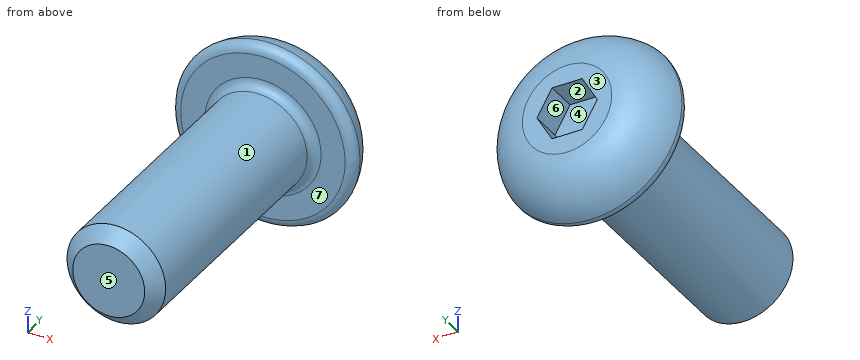
from build123d import *

# Parameters (mm, degrees)
SKETCH2_R           = 1.7526
BOSS_EXTRUDE1_DEPTH = 9.525
CUT_EXTRUDE1_DEPTH  = 1.1176
CHAMFER1_SIZE       = 0.47244
FILLET1_R           = 0.316308646


with BuildPart() as part:
    # Sketch1 → Revolve1 (revolve)
    with BuildSketch(Plane.XY):
        with BuildLine():
            Line((1.5875, 1.8542), (0, 1.8542))
            Line((0, 1.8542), (0, 0))
            Line((0, 0), (3.270560013, 0))
            ThreePointArc((3.270560013, 0), (2.787047666, 1.252073146), (1.5875, 1.8542))
        make_face()
    revolve(axis=Axis((0, 1.8542, 0), (0, -1, 0)))

    # Sketch2 → Boss-Extrude1 (add)
    with BuildSketch(Plane.XZ):
        Circle(SKETCH2_R)
    extrude(amount=BOSS_EXTRUDE1_DEPTH)

    # Sketch3 → Cut-Extrude1 (cut)
    with BuildSketch(Plane(origin=(0, 1.8542, 0), x_dir=(-1, 0, 0), z_dir=(0, 1, 0))):
        Polygon((0.536575, -0.929375162), (1.07315, 0), (0.536575, 0.929375162), (-0.536575, 0.929375162), (-1.07315, 0), (-0.536575, -0.929375162), align=None)
    extrude(amount=-CUT_EXTRUDE1_DEPTH, mode=Mode.SUBTRACT)

    # Chamfer1
    chamfer1_edges = [part.edges().sort_by_distance(p)[0] for p in [
        (-1.7526, -9.525, 0),
    ]]
    chamfer(chamfer1_edges, length=CHAMFER1_SIZE)

    # Fillet1
    fillet1_edges = [part.edges().sort_by_distance(p)[0] for p in [
        (-3.270560013, 0, 0),
        (-1.7526, 0, 0),
    ]]
    fillet(fillet1_edges, radius=FILLET1_R)


solid = part.part
Build history of the part. All positions in model axes, mm. Face numbers are marked on the shaded views. A direction names the side the tool comes from. Give positions to 0.01 mm unless a question says otherwise; leave off trailing zeros. Write each loop counter-clockwise with the first axis right and the second up, starting at its lowest first coordinate (ties: lowest second). Pieces come first, ordered by that corner, then holes. Notation, with made-up numbers: (-3.75, -37.5) - (14.25, -37.5) arc R11 cw to (14.25, -21.5) - close; hole circle Ø4 at (87.5, 79.25). An arc over 180 degrees is marked (long way). Use one line per item in the form item = value. Start each with the question number.
1. Band-saw the part on A-A on y = -2.5. Write the cut outline in (x, z).
2. 3-axis set-ups, long thin cutter, end or side, ignore diameter. For the marked faces 5, 6 and 7: which of +Z, -Z, +X, -X, +Y, -Y reach the whole face in a straight line?
3. Probe line 1 (Z direction, x = 1.25, y = -2.5); line 2 (Z direction, x = 1.25, y = 1.5); line 3 (Y direction, x = 1.5, z = -1.25). List the from-to ranges inside material, lowest first. Write a range as [from, to].
4. Two-plate mould, pull along Z, no slides. Class the marked faces 1, 2, 3 and 4: released by +Z, released by -Z, zero draft, split by the parting line, or undercut.
5. Drop flat-ended pins along their axis: pin 1 Ø0.9 at (x, y) = (0, 1) entering from -Z; pin 2 Ø1.2 at (x, y) = (0, 1.5) entering from +Z. Give the stop position or say it passes through.
Conclusion:
q1.outline = circle Ø3.51 at (0, 0)
q2.face_5 = +Z, -Z, +X, -X, -Y
q2.face_6 = +Y
q2.face_7 = -Y
q3.line_1 = [-1.23, 1.23]
q3.line_2 = [-2.18, 2.18]
q3.line_3 = [-0.02, 1.78]
q4.face_1 = split by the parting line
q4.face_2 = undercut
q4.face_3 = zero draft
q4.face_4 = undercut
q5.pin_1 = -3.19
q5.pin_2 = 3.04
